The model under review builds one solid part; all positions refer to its coordinate system, in mm. Face numbers are marked on the shaded views. A direction names the side the tool comes from. Round coordinates to 2 decimals unless told otherwise and drop trailing zeros. Order: outer loops, then holes, each group sorted by start corner. A loop starts at its lowest first (then second) coordinate and runs counter-clockwise, first axis right, second up. Notation, with made-up numbers: (11.25, 8.5) -> (40.25, 8.5) arc R31 ccw to (40.25, 38.5) -> close; hole circle Ø1 at (65, -27). An arc over 180 degrees is marked (long way). Return JSON: item names as keys, results as strings. Group by question number.
from build123d import *

# Parameters (mm, degrees)
SKETCH1_W           = 20
SKETCH1_H           = 30
BOSS_EXTRUDE1_DEPTH = 3
SKETCH2_W           = 20
SKETCH2_H           = 3
BOSS_EXTRUDE2_DEPTH = 12
SKETCH3_R           = 2.175
CUT_EXTRUDE1_DEPTH  = 12
SKETCH5_R           = 1.725
CUT_EXTRUDE2_DEPTH  = 12
BOSS_EXTRUDE3_DEPTH = 2


with BuildPart() as part:
    # Sketch1 → Boss-Extrude1 (new body)
    with BuildSketch(Plane.XY):
        with Locations((5.222929936, 11.719745223)):
            Rectangle(SKETCH1_W, SKETCH1_H)
    extrude(amount=BOSS_EXTRUDE1_DEPTH)

    # Sketch2 → Boss-Extrude2 (add)
    with BuildSketch(Plane(origin=(0, 0, 0), x_dir=(-1, 0, 0), z_dir=(0, 0, -1))):
        with Locations((-5.222929936, 25.219745223)):
            Rectangle(SKETCH2_W, SKETCH2_H)
    extrude(amount=BOSS_EXTRUDE2_DEPTH)

    # Sketch3 → Cut-Extrude1 (cut)
    with BuildSketch(Plane(origin=(0, 26.719745223, 0), x_dir=(1, 0, 0), z_dir=(0, 1, 0))):
        with Locations(Location((5.222929936, 5, 0), (0, 0, 270))):
            Circle(SKETCH3_R)
    extrude(amount=-CUT_EXTRUDE1_DEPTH, mode=Mode.SUBTRACT)

    # Sketch5 → Cut-Extrude2 (cut)
    with BuildSketch(Plane(origin=(0, 0, 0), x_dir=(-1, 0, 0), z_dir=(0, 0, -1))):
        with Locations((-5.222929936, 6.719745223)):
            Circle(SKETCH5_R)
    extrude(amount=-CUT_EXTRUDE2_DEPTH, mode=Mode.SUBTRACT)

    # Sketch6 → Boss-Extrude3 (add)
    with BuildSketch(Plane.ZY.offset(4.777070064)):
        Polygon((-12, 23.719745223), (0, 23.719745223), (0, 12.719745223), align=None)
    boss_extrude3 = extrude(amount=-BOSS_EXTRUDE3_DEPTH)

    # Mirror1: Boss-Extrude3 across plane
    add(boss_extrude3.mirror(Plane.ZY.offset(-5.222929936)))


solid = part.part
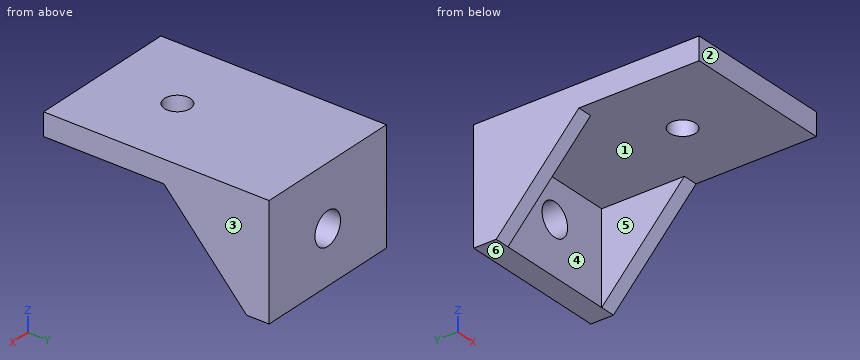
Item 1: Wall thickness on line 1 along X through (y, z) = (25.9, -5); line 2 along X through (y, z) = (21.75, -6.5); line 3 along Z through (x, y) = (4.25, 10.25): over which ranges is each line inside the solid? List them lowest first.
Item 2: Consider section B-B on z = -6.25. State the section outline as (x, y) points.
Item 3: Consider section C-C on x = -0.25. State the section outline as (y, z) points.
Item 4: For the marked faces 1 and 2, list the 3-axis set-ups (+Z, -Z, +X, -X, +Y, -Y) from which the entire face can be reached by the end or side of a thin tool; tool diameter is ignored.
Item 5: The part is to be moulded in two halves that separate along X. For the marked faces 3, 4, 5 and 6, say which applies: +X half, -X half, draft (parallel to the pull), parting line (faces both ways), or undercut.
Item 6: Consider section D-D on y = 16. State the section outline as (x, z) points, plus the area to 3 significant figures.
Item 7: Insertion check: pin 1 Ø2 at (x, y) = (-0.5, 4.5) entering from -Z; pin 2 Ø5 at (x, z) = (5, -6.5) entering from +Y; pin 3 Ø6 at (x, z) = (6, -6) entering from -Y. Each pin has a flat end and moves straight along its axis. Give the tip position at first contact, or say it passes through.
Item 8: Consider section A-A on y = 5.5. State the section outline as (x, z) points, plus the area to 3 significant figures.
Values:
{
 "1": {"line 1": "-4.78 to 3.05, 7.4 to 15.22", "line 2": "-4.78 to -2.78, 13.22 to 15.22", "line 3": "0 to 3"},
 "2": {"outline": "(-4.78, 18.45) -> (-2.78, 18.45) -> (-2.78, 23.72) -> (3.44, 23.72) -> (3.44, 26.72) -> (-4.78, 26.72) -> close; (7, 23.72) -> (13.22, 23.72) -> (13.22, 18.45) -> (15.22, 18.45) -> (15.22, 26.72) -> (7, 26.72) -> close"},
 "3": {"outline": "(-3.28, 0) -> (23.72, 0) -> (23.72, -12) -> (26.72, -12) -> (26.72, 3) -> (-3.28, 3) -> close"},
 "4": {"face 1": "-Z, -Y", "face 2": "+Z, -Z, +X, -X, -Y"},
 "5": {"face 3": "+X half", "face 4": "undercut", "face 5": "undercut", "face 6": "draft"},
 "6": {"outline": "(-4.78, -3.58) -> (-2.78, -3.58) -> (-2.78, 0) -> (13.22, 0) -> (13.22, -3.58) -> (15.22, -3.58) -> (15.22, 3) -> (-4.78, 3) -> close", "area": "74.3 mm^2"},
 "7": {"pin 1": "z = 0", "pin 2": "y = 26.72", "pin 3": "y = 23.72"},
 "8": {"outline": "(-4.78, 0) -> (4, 0) -> (4, 3) -> (-4.78, 3) -> close; (6.44, 0) -> (15.22, 0) -> (15.22, 3) -> (6.44, 3) -> close", "area": "52.7 mm^2"}
}
